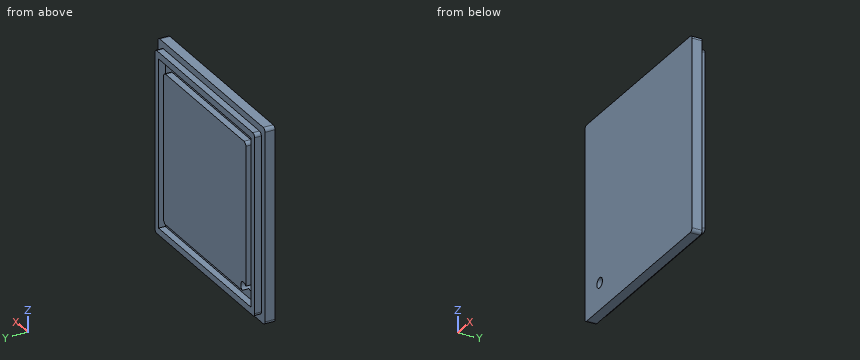
```python
from build123d import *

# Parameters (mm, degrees)
SKETCH005_W   = 54
SKETCH005_H   = 54
SKETCH005_W_2 = 50
SKETCH005_H_2 = 50
SKETCH005_W_3 = 44.5
SKETCH005_H_3 = 44.5
PAD002_DEPTH  = 2
SKETCH006_W   = 58
SKETCH006_H   = 58
PAD003_DEPTH  = 3
FILLET_R      = 1
SKETCH007_R   = 1.5
POCKET_DEPTH  = 5.001


with BuildPart() as part:
    # Sketch005 → Pad002 (new body)
    with BuildSketch(Plane.XZ):
        with Locations((0, 24.25)):
            Rectangle(SKETCH005_W, SKETCH005_H)
        with Locations((0, 24.25)):
            Rectangle(SKETCH005_W_2, SKETCH005_H_2, mode=Mode.SUBTRACT)
        with Locations((0, 24.25)):
            Rectangle(SKETCH005_W_3, SKETCH005_H_3)
    extrude(amount=-PAD002_DEPTH)

    # Sketch006 (on Face15 of Pad002) → Pad003 (join)
    with BuildSketch(Plane.XZ):
        with Locations((0, 24.25)):
            Rectangle(SKETCH006_W, SKETCH006_H)
    extrude(amount=PAD003_DEPTH)

    # Fillet
    fillet_edges = [part.edges().sort_by_distance(p)[0] for p in [
        (-29, -1.5, 53.25),
        (-27, 1, 51.25),
        (-22.25, 1, 46.5),
        (22.25, 1, 46.5),
        (27, 1, 51.25),
        (29, -1.5, 53.25),
        (29, -1.5, -4.75),
        (27, 1, -2.75),
        (22.25, 1, 2),
        (-29, -1.5, -4.75),
        (-27, 1, -2.75),
        (-22.25, 1, 2),
    ]]
    fillet(fillet_edges, radius=FILLET_R)

    # Sketch007 (on Face33 of Fillet) → Pocket (cut, through all)
    with BuildSketch(Plane(origin=(0, 2, 0), x_dir=(1, 0, 0), z_dir=(0, 1, 0))):
        with Locations((-21.008142, -3.295312)):
            Circle(SKETCH007_R)
    extrude(amount=-POCKET_DEPTH, mode=Mode.SUBTRACT)


solid = part.part
```
Part model, mm, in its own coordinate system. Coordinates: 2 decimals unless noted, no trailing zeros. Write each loop counter-clockwise with the first axis right and the second up, starting at its lowest first coordinate (ties: lowest second). Pieces come first, ordered by that corner, then holes.
Item 1: Slice it at A-A (z = 27). Write the cut outline in (x, y), and give its area (3 significant figures).
Item 2: Pin check, flat tips, straight feed: pin 1 (0.6 mm diameter, centred on y = 0.5, z = 17, fed in from -X); pin 2 (1.6 mm diameter, centred on y = 1, z = 33.5, fed in from +X); pin 3 (1 mm diameter, centred on x = -6, y = 1.5, fed in from -Z). Stop position of each tip, or through.
Item 3: Slice it at B-B (x = 16.5). Write the cut outline in (y, z), and give its area (3 significant figures).
Item 4: Probe line 1 (X direction, y = 0.1, z = 5); line 2 (Z direction, x = -18, y = 1.6). List the from-to ranges inside material, lowest first.
Item 5: Slice it at C-C (z = 0). Write the cut outline in (x, y), and give its area (3 significant figures).
Results found:
1. outline: (-29, -3) - (29, -3) - (29, 0) - (27, 0) - (27, 2) - (25, 2) - (25, 0) - (22.25, 0) - (22.25, 2) - (-22.25, 2) - (-22.25, 0) - (-25, 0) - (-25, 2) - (-27, 2) - (-27, 0) - (-29, 0) - close
1. area: 271 mm2
2. pin 1: stops at x = -27
2. pin 2: stops at x = 27
2. pin 3: stops at z = -2.75
3. outline: (-3, -4.75) - (0, -4.75) - (0, -2.75) - (2, -2.75) - (2, -0.75) - (0, -0.75) - (0, 2) - (2, 2) - (2, 46.5) - (0, 46.5) - (0, 49.25) - (2, 49.25) - (2, 51.25) - (0, 51.25) - (0, 53.25) - (-3, 53.25) - close
3. area: 271 mm2
4. line 1: x = -27 to -25, -22.25 to 22.25, 25 to 27
4. line 2: z = -2.75 to -0.75, 2 to 46.5, 49.25 to 51.25
5. outline: (-29, -3) - (29, -3) - (29, 0) - (27, 0) - (27, 2) - (25, 2) - (25, 0) - (-25, 0) - (-25, 2) - (-27, 2) - (-27, 0) - (-29, 0) - close
5. area: 182 mm2
